Could you check a few things on this model? Use its own coordinates, in mm. A direction names the side the tool comes from. Coordinates: 2 decimals unless noted, no trailing zeros. Order: outer loops, then holes, each group sorted by start corner. A loop starts at its lowest first (then second) coordinate and runs counter-clockwise, first axis right, second up.
```python
from build123d import *

# Parameters (mm, degrees)
SKETCH3_R               = 4.5
BOSS_EXTRUDE3_DEPTH     = 6.5
SKETCH4_R               = 3
CUT_EXTRUDE1_DEPTH      = 2.5
SKETCH5_R               = 2
CUT_EXTRUDE2_DEPTH      = 1.95
CUT_EXTRUDE3_REACH      = 11.097
CUT_EXTRUDE3_END_RADIUS = 4.5
SKETCH7_R               = 0.825


with BuildPart() as part:
    # Sketch3 → Boss-Extrude3 (new body)
    with BuildSketch(Plane.XY):
        with Locations(Location((0, 0, 0), (0, 0, 180))):
            Circle(SKETCH3_R)
    extrude(amount=BOSS_EXTRUDE3_DEPTH)

    # Sketch4 → Cut-Extrude1 (cut)
    with BuildSketch(Plane.XY.offset(6.5)):
        Circle(SKETCH4_R)
    extrude(amount=-CUT_EXTRUDE1_DEPTH, mode=Mode.SUBTRACT)

    # Sketch5 → Cut-Extrude2 (cut)
    with BuildSketch(Plane(origin=(0, 0, 0), x_dir=(-1, 0, 0), z_dir=(0, 0, -1))):
        Circle(SKETCH5_R)
    extrude(amount=-CUT_EXTRUDE2_DEPTH, mode=Mode.SUBTRACT)

    # Cut-Extrude3: up to this cylinder (the profile starts inside it)
    cut_extrude3_end = Plane(origin=(0, 0, 5.2), z_dir=(0, 0, -1)) * Cylinder(CUT_EXTRUDE3_END_RADIUS, 32.194, mode=Mode.PRIVATE)
    # Sketch7 → Cut-Extrude3 (cut, up to the surface)
    with BuildSketch(Plane(origin=(0, 0, 0), x_dir=(1, 0, 0), z_dir=(0, 1, 0)), mode=Mode.PRIVATE) as cut_extrude3_sk1:
        with Locations(Location((0, -5.2, 0), (0, 0, 270))):
            Circle(SKETCH7_R)
    cut_extrude3_tool1 = extrude(cut_extrude3_sk1.sketch, amount=-CUT_EXTRUDE3_REACH, mode=Mode.PRIVATE) & cut_extrude3_end
    add(cut_extrude3_tool1.solids().sort_by_distance((0, 0, 5.2))[0], mode=Mode.SUBTRACT)


solid = part.part
```
Item 1: Suppose I cut it at B-B (z = 6.25). List the corners of the cut face in (x, y) for me.
Item 2: Suppose I cut it at A-A (x = 0). List the corners of the cut face in (y, z) for me (3 decimals), and give its area (3 significant figures).
Item 3: Thinking about a two-plate mould opening in Y: for faces 4 (the face through (0, 0, 1.95)), 5 (the face through (-2, 1, 0)), 6 (the face through (0.98, 4.39, 3.2)), which applies, +Y half, -Y half, draft (parallel to the pull), parting line (faces both ways), or undercut?
Item 4: Suppose I cut it at C-C (y = -1.5). List the corners of the cut face in (x, z) for me.
Item 5: Which directions (+Z, -Z, +X, -X, +Y, -Y) give clear straight access to the entire face, cutting with the end or side of a thin tool? Please do faces 1 (the face through (0, 3, 5)), 2 (the face through (0, -2, 1)), 3 (the face through (0.036, -3.681, 4.376)).
Item 6: For pin 1 Ø2.5 at (x, z) = (0, 5.2) entering from -Y; pin 2 Ø3 at (y, z) = (-2.5, 4.5) entering from +X; pin 3 Ø3 at (x, z) = (-3.5, 5) entering from -Y; pin 4 Ø3.5 at (x, y) = (0, 0) entering from -Z, each with a flat end and sliding along its axis, tell me the tip position at first contact or that it passes through.
Item 7: I need wall thicknesses on line 1 (Y direction, x = 0, z = 1.3); line 2 (Z direction, x = 0, y = -3.25) (3 decimals); line 3 (Z direction, x = -2, y = -0.75). Which ranges of each line are inside material? Lowest first, please.
Geometry results:
1. outline: circle Ø9 at (0, 0); hole circle Ø6 at (0, 0)
2. outline: (-4.5, 0) - (-2, 0) - (-2, 1.95) - (2, 1.95) - (2, 0) - (4.5, 0) - (4.5, 6.5) - (3, 6.5) - (3, 4) - (-3, 4) - (-3, 4.375) - (-4.5, 4.375) - close; (-4.5, 6.025) - (-3, 6.025) - (-3, 6.5) - (-4.5, 6.5) - close
2. area: 33.2 mm2
3. face 4: undercut
3. face 5: draft
3. face 6: parting line
4. outline: (-4.24, 0) - (-1.32, 0) - (-1.32, 1.95) - (1.32, 1.95) - (1.32, 0) - (4.24, 0) - (4.24, 6.5) - (2.6, 6.5) - (2.6, 4) - (-2.6, 4) - (-2.6, 6.5) - (-4.24, 6.5) - close
5. face 1: +Z
5. face 2: -Z
5. face 3: -Y
6. pin 1: stops at y = -4.5
6. pin 2: stops at x = 4.39
6. pin 3: stops at y = -4.03
6. pin 4: stops at z = 1.95
7. line 1: y = -4.5 to -2, 2 to 4.5
7. line 2: z = 0 to 4.375, 6.025 to 6.5
7. line 3: z = 0 to 4
